from build123d import *

# Parameters (mm, degrees)
SKETCH1_R           = 4
SKETCH1_R_2         = 1.5
BOSS_EXTRUDE1_DEPTH = 3
SKETCH2_R           = 3.653156204
SKETCH2_R_2         = 1.91674474
CUT_EXTRUDE1_DEPTH  = 0.1
SKETCH4_R           = 2.048114098
SKETCH4_R_2         = 1.91674474
CUT_EXTRUDE6_DEPTH  = 0.1
SKETCH5_R           = 3.653156204
SKETCH5_R_2         = 3.522114118
CUT_EXTRUDE7_DEPTH  = 0.1
SKETCH6_R           = 3.611227951
CUT_EXTRUDE8_DEPTH  = 2.1


with BuildPart() as part:
    # Sketch1 → Boss-Extrude1 (new body)
    with BuildSketch(Plane(origin=(0, 0, 0), x_dir=(1, 0, 0), z_dir=(0, 1, 0))):
        Circle(SKETCH1_R)
        Circle(SKETCH1_R_2, mode=Mode.SUBTRACT)
    extrude(amount=BOSS_EXTRUDE1_DEPTH)

    # Sketch2 → Cut-Extrude1 (cut)
    with BuildSketch(Plane(origin=(0, 3, 0), x_dir=(1, 0, 0), z_dir=(0, 1, 0))):
        Circle(SKETCH2_R)
        Circle(SKETCH2_R_2, mode=Mode.SUBTRACT)
    extrude(amount=-CUT_EXTRUDE1_DEPTH, mode=Mode.SUBTRACT)

    # Sketch4 → Cut-Extrude6 (cut)
    with BuildSketch(Plane(origin=(0, 2.9, 0), x_dir=(1, 0, 0), z_dir=(0, 1, 0))):
        Circle(SKETCH4_R)
        Circle(SKETCH4_R_2, mode=Mode.SUBTRACT)
    extrude(amount=-CUT_EXTRUDE6_DEPTH, mode=Mode.SUBTRACT)

    # Sketch5 → Cut-Extrude7 (cut)
    with BuildSketch(Plane(origin=(0, 2.9, 0), x_dir=(1, 0, 0), z_dir=(0, 1, 0))):
        Circle(SKETCH5_R)
        Circle(SKETCH5_R_2, mode=Mode.SUBTRACT)
    extrude(amount=-CUT_EXTRUDE7_DEPTH, mode=Mode.SUBTRACT)

    # Sketch6 → Cut-Extrude8 (cut)
    with BuildSketch(Plane.XZ):
        Circle(SKETCH6_R)
    extrude(amount=-CUT_EXTRUDE8_DEPTH, mode=Mode.SUBTRACT)


solid = part.part
Geometry: final body of the model. Coordinates: model frame, mm. A direction names the side the tool comes from. Round coordinates to 2 decimals unless told otherwise and drop trailing zeros. Order: outer loops, then holes, each group sorted by start corner. A loop starts at its lowest first (then second) coordinate and runs counter-clockwise, first axis right, second up.
Q1. Access query for faces 1 (the face through (2, 2.9, 2)), 2 (the face through (3.444, 1.035, 1.085)). Directions: +Z, -Z, +X, -X, +Y, -Y. A direction counts if a zero-diameter tool reaches every point of the face in a straight line with its end or side. Return the directions, or none.
Result sheet:
face 1: +Y
face 2: -Y
Q2. Section A-A, the plane x = 0. Output: boundary loops of the cut face in (y, z).
Result sheet:
outline: (0, -4) - (3, -4) - (3, -3.65) - (2.8, -3.65) - (2.8, -3.52) - (2.9, -3.52) - (2.9, -2.05) - (2.8, -2.05) - (2.8, -1.92) - (3, -1.92) - (3, -1.5) - (2.1, -1.5) - (2.1, -3.61) - (0, -3.61) - close; (0, 3.61) - (2.1, 3.61) - (2.1, 1.5) - (3, 1.5) - (3, 1.92) - (2.8, 1.92) - (2.8, 2.05) - (2.9, 2.05) - (2.9, 3.52) - (2.8, 3.52) - (2.8, 3.65) - (3, 3.65) - (3, 4) - (0, 4) - close
Q3. Pin query (flat end, axial travel): pin 1 (2 mm diameter, centred on x = -0.5, z = 0.5, fed in from +Y); pin 2 (2 mm diameter, centred on x = 1.5, z = 0.5, fed in from -Y). Return the tip coordinate at first contact, or that it passes through.
Result sheet:
pin 1: stops at y = 3
pin 2: stops at y = 2.1
Q4. Section B-B, the plane z = 0. Output: boundary loops of the cut face in (x, y), and give its area (3 significant figures).
Result sheet:
outline: (-4, 0) - (-3.61, 0) - (-3.61, 2.1) - (-1.5, 2.1) - (-1.5, 3) - (-1.92, 3) - (-1.92, 2.8) - (-2.05, 2.8) - (-2.05, 2.9) - (-3.52, 2.9) - (-3.52, 2.8) - (-3.65, 2.8) - (-3.65, 3) - (-4, 3) - close; (1.5, 2.1) - (3.61, 2.1) - (3.61, 0) - (4, 0) - (4, 3) - (3.65, 3) - (3.65, 2.8) - (3.52, 2.8) - (3.52, 2.9) - (2.05, 2.9) - (2.05, 2.8) - (1.92, 2.8) - (1.92, 3) - (1.5, 3) - close
area: 5.73 mm2
Q5. Section D-D, the plane z = 2.25. Output: boundary loops of the cut face in (x, y).
Result sheet:
outline: (-3.31, 0) - (-2.82, 0) - (-2.82, 2.1) - (2.82, 2.1) - (2.82, 0) - (3.31, 0) - (3.31, 3) - (2.88, 3) - (2.88, 2.8) - (2.71, 2.8) - (2.71, 2.9) - (-2.71, 2.9) - (-2.71, 2.8) - (-2.88, 2.8) - (-2.88, 3) - (-3.31, 3) - close
Q6. Mould query, pull axis Z, two halves, no side actions, for faces 3 (the face through (-1.5, 2.54, -0.07)), 4 (the face through (0, 2.1, -2)), 5 (the face through (-0.867, 1.479, 3.905)). Classes: released by +Z, released by -Z, zero draft, split by the parting line, or undercut.
Result sheet:
face 3: undercut
face 4: undercut
face 5: split by the parting line
Q7. Material intervals for probe 1 along Z at (x, y) = (0, 2.95); probe 2 along Z at (x, y) = (0, 1.2), sorted ascending.
Result sheet:
probe 1: z = -4 to -3.65, -1.92 to -1.5, 1.5 to 1.92, 3.65 to 4
probe 2: z = -4 to -3.61, 3.61 to 4
Q8. Section C-C, the plane y = 0.25. Output: boundary loops of the cut face in (x, z), and give its area (3 significant figures).
Result sheet:
outline: circle Ø8 at (0, 0); hole circle Ø7.22 at (0, 0)
area: 9.30 mm2
